```python
from build123d import *

# Parameters (mm, degrees)
CUT_EXTRUDE1_REACH = 42
SKETCH2_R          = 4
CHAMFER1_SIZE      = 0.75


with BuildPart() as part:
    # Sketch1 → Revolve1 (revolve)
    with BuildSketch(Plane.XY):
        Polygon((-24.15, 5.519256014), (-24.15, -34.480743986), (-30, -34.480743986), (-30, -6.480743986), (-36, -6.480743986), (-36, -4.480743986), (-79, -4.480743986), (-79, 5.519256014), align=None)
    revolve(axis=Axis((0, 0, 0), (0, -1, 0)))

    # Sketch2 → Cut-Extrude1 (cut, up to next)
    with BuildSketch(Plane(origin=(0, 5.519256014, 0), x_dir=(1, 0, 0), z_dir=(0, 1, 0)), mode=Mode.PRIVATE) as cut_extrude1_sk1:
        with Locations((48.790367902, 48.790367902)):
            Circle(SKETCH2_R)
    cut_extrude1_tool1 = extrude(cut_extrude1_sk1.sketch, amount=-CUT_EXTRUDE1_REACH, mode=Mode.PRIVATE) & part.part
    add(cut_extrude1_tool1.solids().sort_by_distance((48.790368, 5.519256, -48.790368))[0], mode=Mode.SUBTRACT)
    # Sketch2 → Cut-Extrude1 (cut, up to next)
    with BuildSketch(Plane(origin=(0, 5.519256014, 0), x_dir=(1, 0, 0), z_dir=(0, 1, 0)), mode=Mode.PRIVATE) as cut_extrude1_sk2:
        with Locations((48.790367902, -48.790367902)):
            Circle(SKETCH2_R)
    cut_extrude1_tool2 = extrude(cut_extrude1_sk2.sketch, amount=-CUT_EXTRUDE1_REACH, mode=Mode.PRIVATE) & part.part
    add(cut_extrude1_tool2.solids().sort_by_distance((48.790368, 5.519256, 48.790368))[0], mode=Mode.SUBTRACT)
    # Sketch2 → Cut-Extrude1 (cut, up to next)
    with BuildSketch(Plane(origin=(0, 5.519256014, 0), x_dir=(1, 0, 0), z_dir=(0, 1, 0)), mode=Mode.PRIVATE) as cut_extrude1_sk3:
        with Locations((-48.790367902, -48.790367902)):
            Circle(SKETCH2_R)
    cut_extrude1_tool3 = extrude(cut_extrude1_sk3.sketch, amount=-CUT_EXTRUDE1_REACH, mode=Mode.PRIVATE) & part.part
    add(cut_extrude1_tool3.solids().sort_by_distance((-48.790368, 5.519256, 48.790368))[0], mode=Mode.SUBTRACT)
    # Sketch2 → Cut-Extrude1 (cut, up to next)
    with BuildSketch(Plane(origin=(0, 5.519256014, 0), x_dir=(1, 0, 0), z_dir=(0, 1, 0)), mode=Mode.PRIVATE) as cut_extrude1_sk4:
        with Locations((-48.790367902, 48.790367902)):
            Circle(SKETCH2_R)
    cut_extrude1_tool4 = extrude(cut_extrude1_sk4.sketch, amount=-CUT_EXTRUDE1_REACH, mode=Mode.PRIVATE) & part.part
    add(cut_extrude1_tool4.solids().sort_by_distance((-48.790368, 5.519256, -48.790368))[0], mode=Mode.SUBTRACT)

    # Chamfer1
    chamfer1_edges = [part.edges().sort_by_distance(p)[0] for p in [
        (79, 5.519256014, 0),
        (79, -4.480743986, 0),
        (30, -34.480743986, 0),
        (24.15, -34.480743986, 0),
        (24.15, 5.519256014, 0),
    ]]
    chamfer(chamfer1_edges, length=CHAMFER1_SIZE)


solid = part.part
```
Source: CAD feature listing. Evaluate the final solid. Frame: model axes, mm. A direction names the side the tool comes from. Give positions to 0.01 mm unless a question says otherwise; leave off trailing zeros. Write each loop counter-clockwise with the first axis right and the second up, starting at its lowest first coordinate (ties: lowest second). Pieces come first, ordered by that corner, then holes.
1. Section query B-B (z = 0). Return the cut outline in (x, y), then the cut area to 3 significant figures.
2. First-contact query: pin 1 (12 mm diameter, centred on x = 34.5, z = 42.5, fed in from -Y); pin 2 (3 mm diameter, centred on y = -28, z = 24, fed in from +X); pin 3 (2 mm diameter, centred on x = -23, y = -25, fed in from +Z). Flat tips, straight axial feed; report the tip coordinate or a pass-through.
3. Access query for faces 4 (the face through (29.97, -19.91, -1.32)), 5 (the face through (52.485, 0.589, -47.258)). Directions: +Z, -Z, +X, -X, +Y, -Y. A direction counts if a zero-diameter tool reaches every point of the face in a straight line with its end or side. Return the directions, or none.
4. Pull-direction query (Z, two-part tool) for faces 1 (the face through (4.686, -5.467, -35.694)), 2 (the face through (22, -34.481, -13)), 3 (the face through (24.127, -14.75, -1.062)); classes: +Z half, -Z half, draft (parallel to the pull), parting line (faces both ways), or undercut.
5. Section query A-A (x = 0). Return the cut outline in (y, z).
6. Material intervals for line 1 along X through (y, z) = (-19.5, 0); line 2 along Z through (x, y) = (-51, -1.5); line 3 along X through (y, z) = (-3, 0), sorted ascending.
7. Section query C-C (y = -29). Return the cut outline in (x, z), then the cut area to 3 significant figures.
Output values:
1. outline: (-79, -3.73) - (-78.25, -4.48) - (-36, -4.48) - (-36, -6.48) - (-30, -6.48) - (-30, -33.73) - (-29.25, -34.48) - (-24.9, -34.48) - (-24.15, -33.73) - (-24.15, 4.77) - (-24.9, 5.52) - (-78.25, 5.52) - (-79, 4.77) - close; (24.15, -33.73) - (24.9, -34.48) - (29.25, -34.48) - (30, -33.73) - (30, -6.48) - (36, -6.48) - (36, -4.48) - (78.25, -4.48) - (79, -3.73) - (79, 4.77) - (78.25, 5.52) - (24.9, 5.52) - (24.15, 4.77) - close
1. area: 1,470 mm2
2. pin 1: stops at y = -4.48
2. pin 2: stops at x = 19.84
2. pin 3: stops at z = 20.4
3. face 4: -Y
3. face 5: +Y, -Y
4. face 1: parting line
4. face 2: draft
4. face 3: undercut
5. outline: (-34.48, -29.25) - (-33.73, -30) - (-6.48, -30) - (-6.48, -36) - (-4.48, -36) - (-4.48, -78.25) - (-3.73, -79) - (4.77, -79) - (5.52, -78.25) - (5.52, -24.9) - (4.77, -24.15) - (-33.73, -24.15) - (-34.48, -24.9) - close; (-34.48, 24.9) - (-33.73, 24.15) - (4.77, 24.15) - (5.52, 24.9) - (5.52, 78.25) - (4.77, 79) - (-3.73, 79) - (-4.48, 78.25) - (-4.48, 36) - (-6.48, 36) - (-6.48, 30) - (-33.73, 30) - (-34.48, 29.25) - close
6. line 1: x = -30 to -24.15, 24.15 to 30
6. line 2: z = -60.33 to -52.12, -45.46 to 45.46, 52.12 to 60.33
6. line 3: x = -79 to -24.15, 24.15 to 79
7. outline: circle Ø60 at (0, 0); hole circle Ø48.3 at (0, 0)
7. area: 995 mm2
